Answer from the drawing. Dimensions are ordinates in mm from the lowest x, y and z of the part. A direction names the side the tool comes from. Round coordinates to 2 decimals unless told otherwise and drop trailing zeros. Loops run counter-clockwise (first coordinate to the right, second up) from the corner with the lowest first, then second, coordinate; pieces in that order, holes last. Notation, with made-up numbers: (1.25, 46) -> (5.25, 46) arc R29 cw to (5.25, 76) -> close; hole circle Ø11 at (80.5, -26). An arc over 180 degrees is marked (long way). One line per question, with ' | ' between items.
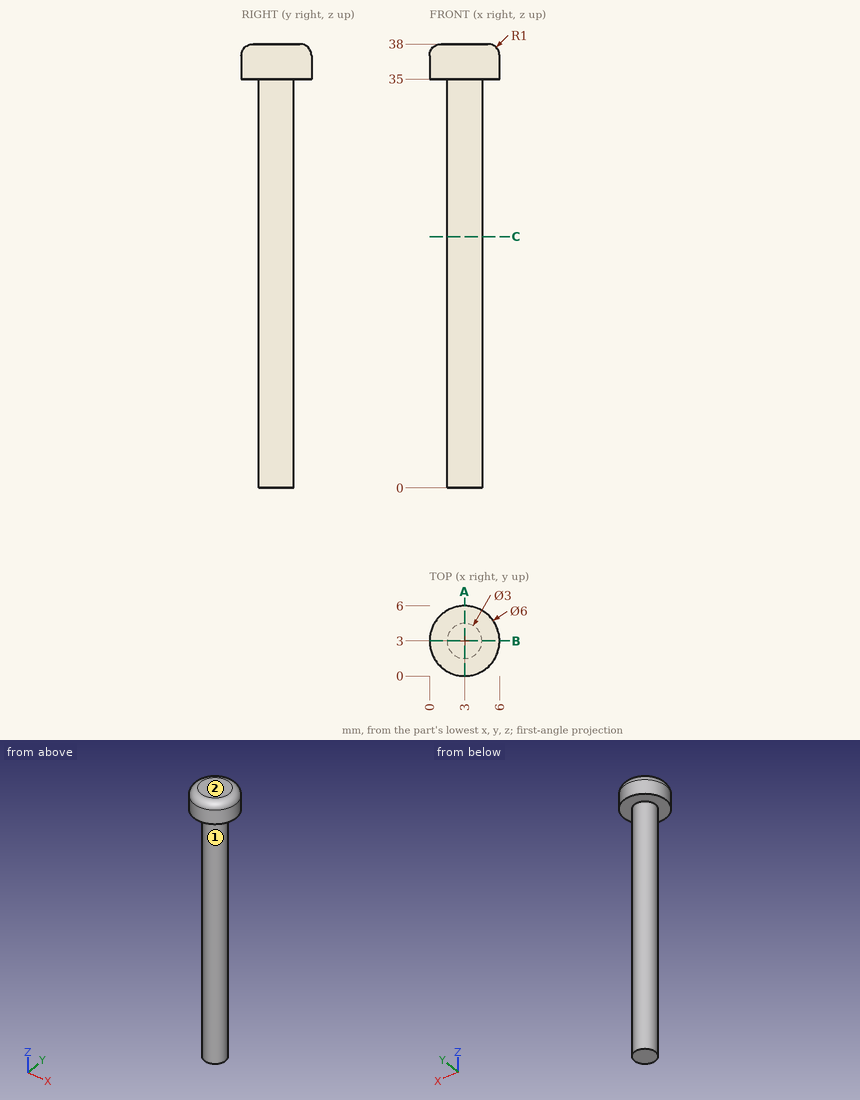
Q1. Find the intervals of material crossed by line 1 (Z direction, x = 4.65, y = 4.25); line 2 (Y direction, x = 3.15, z = 6.5); line 3 (Y direction, x = 3.7, z = 36), in increasing order. Write a range as from..to.
Numbers:
line 1: 35..38 | line 2: 1.51..4.49 | line 3: 0.08..5.92
Q2. For the marked faces 1 and 2, determine the directions among +Z, -Z, +X, -X, +Y, -Y from which every point of the face is accessible in a straight line to the end or side of a thin tool.
Numbers:
face 1: -Z | face 2: +Z, +X, -X, +Y, -Y
Q3. Given pin 1 Ø1.5 at (x, z) = (4, 4.5) entering from -Y; pin 2 Ø1 at (x, y) = (5, 1) entering from +Z, each flat-ended and moving along its own axis, determine where each tip first touches the part or whether it passes through.
Numbers:
pin 1: y = 1.52 | pin 2: z = 37.94
Q4. A cutting plane is placed at A-A on x = 3. Give the vertices of the cut face in (y, z).
Numbers:
outline: (0, 35) -> (1.5, 35) -> (1.5, 0) -> (4.5, 0) -> (4.5, 35) -> (6, 35) -> (6, 37) arc R1 ccw to (5, 38) -> (1, 38) arc R1 ccw to (0, 37) -> close
Q5. A cutting plane is placed at C-C on z = 21.5. Give the vertices of the cut face in (x, y), plus the area to 3 significant figures.
Numbers:
outline: circle Ø3 at (3, 3) | area: 7.07 mm^2
